Autodesk Inventor part; units mm, degrees
ref_plane "YZ Plane" through (0, 0, 0) normal (1, 0, 0) x (0, 1, 0)
ref_plane "XZ Plane" through (0, 0, 0) normal (0, 1, 0) x (-1, 0, 0)
ref_plane "XY Plane" through (0, 0, 0) normal (0, 0, 1) x (1, 0, 0)
sketch "草圖1" plane through (0, 0, 0) normal (0, 1, 0) x (-1, 0, 0)
  line L0 (5.5, -3) -> (-5.5, -3)
  line L1 (-5.5, -3) -> (-5.5, -15.75)
  line L2 (-5.5, -15.75) -> (5.5, -15.75)
  line L3 (5.5, -15.75) -> (5.5, -3)
  line L4 (-9, -39.5104) -> (-5, -39.5058)
  line L5 (-5, -39.5058) -> (-4.9985, -40.8058)
  line L6 (-4.9985, -40.8058) -> (-1.9985, -40.8023)
  line L7 (-1.9985, -40.8023) -> (-2, -39.5023)
  line L8 (-2, -39.5023) -> (0, -39.5)
  line L9 (-5, -35.2) -> (-2, -35.2)
  line L10 (-5, -36.5) -> (-5, -35.2)
  line L11 (-2, -35.2) -> (-2, -36.5)
  line L12 (-2, -36.5) -> (0, -36.5)
  line L13 (-9, -36.5) -> (-5, -36.5)
  line L14 (-12, 0) -> (-12, -5)
  line L15 (-12, -5) -> (-9, -5)
  line L16 (-9, -5) -> (-9, -36.5)
  line L17 (-12, 0) -> (-12, -5)
  line L18 (11.9851, -47) -> (8.9851, -47)
  line L19 (7.5982, -47) -> (9.4378, -47)
  arc A0 (7.5982, -47) -> (4.5816, -50.0166) centre (7.5982, -50.0166) ccw
  line L20 (0, -36.5) -> (0, -39.5)
  line L21 (-12, 0) -> (-12, -5)
  line L22 (-12, -5) -> (-9, -5)
  line L23 (-9, -5) -> (-9, -36.5)
  line L24 (-9, -36.5) -> (-5, -36.5)
  line L25 (-5, -36.5) -> (-5, -35.2)
  line L26 (-5, -35.2) -> (-2.2106, -35.2)
  line L27 (-5, -35.2) -> (-2, -35.2)
  line L28 (-2, -35.2) -> (-2, -36.5)
  line L29 (-2, -36.5) -> (0, -36.5)
  line L30 (0, -36.5) -> (0, -39.5)
  line L31 (0, -39.5) -> (-2, -39.5023)
  line L32 (-2, -39.5023) -> (-1.9985, -40.8023)
  line L33 (-1.9985, -40.8023) -> (-4.9985, -40.8058)
  line L34 (-4.9985, -40.8023) -> (-5, -39.5058)
  line L35 (-5, -39.5058) -> (-9, -39.5104)
  line L36 (-9, -39.5104) -> (-9, -52.5104)
  line L37 (-9, -52.5104) -> (-12.0184, -52.5104)
  line L38 (11.9851, -47) -> (7.5982, -47)
  line L39 (11.985, -7.9789) -> (11.985, 0)
  line L40 (11.985, 0) -> (-12, 0)
  line L41 (11.985, -7.9789) -> (8.985, -7.9789)
  line L42 (8.985, -7.9789) -> (8.985, -20.4789)
  line L43 (8.9851, -38) -> (11.9851, -38)
  line L44 (8.985, -20.4789) -> (4.985, -20.4789)
  line L45 (4.985, -20.4789) -> (4.985, -19.1789)
  line L46 (4.985, -19.1789) -> (1.985, -19.1789)
  line L47 (1.985, -19.1789) -> (1.985, -20.4789)
  line L48 (1.985, -20.4789) -> (-0.015, -20.4789)
  line L49 (-0.015, -20.4789) -> (-0.015, -23.4789)
  line L50 (1.985, -23.4789) -> (-0.015, -23.4789)
  line L51 (1.985, -23.4789) -> (1.985, -24.7789)
  line L52 (4.985, -24.7789) -> (1.985, -24.7789)
  line L53 (4.985, -24.7789) -> (4.985, -23.4789)
  line L54 (4.985, -23.5) -> (8.9851, -23.5)
  line L55 (8.9851, -23.5) -> (8.9851, -38)
  line L56 (11.9851, -38) -> (11.9851, -47)
  line L57 (4.5816, -50.0166) -> (4.5816, -60)
  line L58 (4.5816, -60) -> (-12.0184, -60)
  line L59 (-12.0184, -52.5104) -> (-12.0184, -60)
  point P0 (0, 0)
  dimension "d2" = 11
  dimension "d3" = 12.75
  dimension "d7" = 3
  dimension "d10" = 4
  dimension "d12" = 3
  dimension "d17" = 4
  dimension "d18" = 1.3
  dimension "d19" = 3
  dimension "d20" = 1.3
  dimension "d21" = 2
  dimension "d22" = 5
  dimension "d23" = 3
  dimension "d25" = 31.5
  dimension "d26" = 13
  dimension "d27" = 14.5
  dimension "d29" = 16.6
  dimension "d30" = 2
extrude "擠出1" add sketch "草圖1" along normal mid plane 3
properties part number "板子10"
Verification items for the finished model (mm, model axes). A direction names the side the tool comes from. Coordinates: 2 decimals unless noted, no trailing zeros. Write each loop counter-clockwise with the first axis right and the second up, starting at its lowest first coordinate (ties: lowest second). Pieces come first, ordered by that corner, then holes. Notation, with made-up numbers: (68.5, 33.5) - (109.5, 33.5) arc R28 ccw to (109.5, 65.5) - close; hole circle Ø10 at (-32, 26.25). An arc over 180 degrees is marked (long way). One line per question, with ' | ' between items. Start each with the question number.
1. Section check D-D (z = -41.5). Enter the section's corners in (x, y), plus the area to 3 significant figures.
2. Gauge pin test, flat ends, axial feed: P1, Ø0.7, axis at y = -0.5, z = -24, coming from the -X side; P2, Ø0.9, axis at x = -10, y = 0, coming from the +Z side; P3, Ø1.5, axis at y = 1, z = -38, coming from the +X side; P4, Ø6, axis at x = -8, z = -53, coming from the +Y side. Record the tip position at first contact, or that the pin passes through.
3. Section check C-C (z = -51.5). Enter the section's corners in (x, y).
4. Section check A-A (z = -13). Enter the section's corners in (x, y) (3 decimals).
5. Access from +Z, -Z, +X, -X, +Y, -Y to the whole of each face (thin tool, end or side, straight path). Record for faces 4 (the flat face through (-11, 0, -7.979)), 5 (the flat face through (-10, 0, -47)), 6 (the flat face through (7, 0, -36.5)), 7 (the flat face through (2, 0, -36)).
6. Section check B-B (x = 2.75). Enter the section's corners in (y, z), plus the area to 3 significant figures.
7. Draft check along X on faces 1 (the flat face through (4, 0, -35.2)), 2 (the flat face through (9, 0, -21)), 3 (the flat face through (1, 0, -36.5)). Enter one of: released by +X, released by -X, zero draft, split by the parting line, or undercut.
8. Material ranges on line 1 along Z through (x, y) = (0.75, 0.5); line 2 along X through (y, z) = (-0.15, -10) (3 decimals); line 3 along Z through (x, y) = (-10, -1.1), recorded low to high.
Computed values:
1) outline: (-11.99, -1.5) - (9, -1.5) - (9, 1.5) - (-11.99, 1.5) - close | area: 63.0 mm²
2) P1: x = -8.99 | P2: z = 0 | P3: x = 0 | P4: through
3) outline: (-4.58, -1.5) - (9, -1.5) - (9, 1.5) - (-4.58, 1.5) - close
4) outline: (-8.985, -1.5) - (-5.5, -1.5) - (-5.5, 1.5) - (-8.985, 1.5) - close; (5.5, -1.5) - (9, -1.5) - (9, 1.5) - (5.5, 1.5) - close
5) face 4: -X, +Y, -Y | face 5: -Z, -X, +Y, -Y | face 6: +X, +Y, -Y | face 7: +Y, -Y
6) outline: (-1.5, -60) - (1.5, -60) - (1.5, -40.8) - (-1.5, -40.8) - close; (-1.5, -35.2) - (1.5, -35.2) - (1.5, -15.75) - (-1.5, -15.75) - close; (-1.5, -3) - (1.5, -3) - (1.5, 0) - (-1.5, 0) - close | area: 125 mm²
7) face 1: undercut | face 2: released by +X | face 3: zero draft
8) line 1: -60 to -39.5, -36.5 to -15.75, -3 to 0 | line 2: -8.985 to -5.5, 5.5 to 9 | line 3: -47 to -38, -7.98 to 0
